Source: CAD feature listing. Evaluate the final solid. Frame: model axes, mm. Face numbers are marked on the shaded views. A direction names the side the tool comes from. Round coordinates to 2 decimals unless told otherwise and drop trailing zeros. Loops run counter-clockwise (first coordinate to the right, second up) from the corner with the lowest first, then second, coordinate; pieces in that order, holes last. Notation, with made-up numbers: (15, 49) -> (40, 49) arc R16 ccw to (40, 66) -> close; hole circle Ø3 at (-8, 50). An arc over 180 degrees is marked (long way). Return JSON: item names as keys, results as strings. Group by question number.
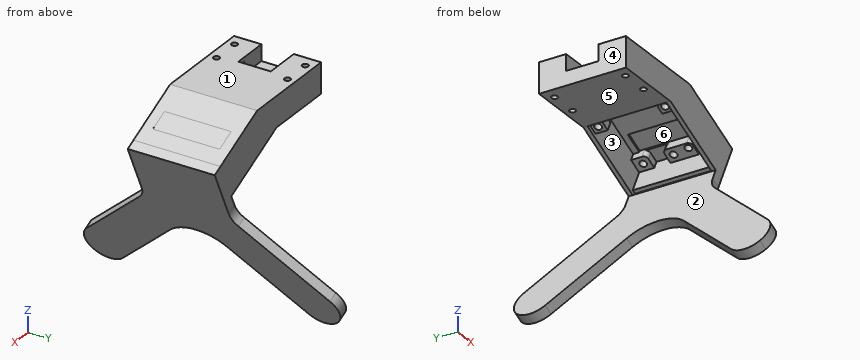
```python
from build123d import *

# Parameters (mm, degrees)
AUFSATZ_LINEAR_AUSTRAGEN1_DEPTH      = 43
AUFSATZ_LINEAR_AUSTRAGEN2_DEPTH      = 5
SCHNITT_LINEAR_AUSTRAGEN1_REACH      = 157.451
SKIZZE3_R                            = 1.5
SKIZZE4_W                            = 8
SKIZZE4_H                            = 16
SCHNITT_LINEAR_AUSTRAGEN2_DEPTH      = 18
SKIZZE5_W                            = 30
SKIZZE5_H                            = 39
SCHNITT_LINEAR_AUSTRAGEN3_DEPTH      = 18
SKIZZE6_W                            = 7
SKIZZE6_H                            = 7.5
SKIZZE6_H_2                          = 14
SKIZZE6_H_3                          = 5.5
AUFSATZ_LINEAR_AUSTRAGEN3_DEPTH      = 4
VERRUNDUNG1_R                        = 2
F_3_4_3_4_DURCHMESSER_BOHRUNG1_D     = 3.4
F_3_4_3_4_DURCHMESSER_BOHRUNG1_DEPTH = 4
SKIZZE10_W                           = 10
SKIZZE10_H                           = 33
SCHNITT_LINEAR_AUSTRAGEN4_DEPTH      = 1
SKIZZE11_W                           = 10
SKIZZE11_H                           = 33
SCHNITT_LINEAR_AUSTRAGEN5_DEPTH      = 0.001
SCHNITT_LINEAR_AUSTRAGEN7_DEPTH      = 39
SKIZZE15_W                           = 10.432594073
SKIZZE15_H                           = 24
SCHNITT_LINEAR_AUSTRAGEN10_DEPTH     = 16
SKIZZE16_W                           = 2.1
SKIZZE16_H                           = 39
SCHNITT_LINEAR_AUSTRAGEN11_DEPTH     = 2
VERRUNDUNG2_R                        = 20
VERRUNDUNG3_R                        = 10
SKIZZE17_W                           = 6
SKIZZE17_H                           = 6
AUFSATZ_LINEAR_AUSTRAGEN4_DEPTH      = 5
FASE1_SIZE                           = 6
F_3_4_3_4_DURCHMESSER_BOHRUNG2_D     = 3.4
F_3_4_3_4_DURCHMESSER_BOHRUNG2_DEPTH = 5
F_3_4_3_4_DURCHMESSER_BOHRUNG2_TIP   = 1.021463052


with BuildPart() as part:
    # Skizze1 → Aufsatz-Linear austragen1 (new body)
    with BuildSketch(Plane(origin=(0, 0, 0), x_dir=(1, 0, 0), z_dir=(0, 1, 0))):
        Polygon((0, 0), (50, 0), (78.641941074, 13.355956467), (70.189575839, 31.482112208), (34.843572145, 15), (0, 15), align=None)
    extrude(amount=AUFSATZ_LINEAR_AUSTRAGEN1_DEPTH)

    # Skizze2 → Aufsatz-Linear austragen2 (add)
    with BuildSketch(Plane(origin=(69.711631316, 0, -32.507067545), x_dir=(-0.4226182617407004, 0, -0.9063077870366495), z_dir=(0.9063077870366495, 0, -0.4226182617407004))):
        Polygon((-21.130913087, 43), (8.869086913, 43), (54.544231126, 88.675144213), (68.686366749, 74.533008589), (15.65335816, 21.5), (68.686366749, -31.533008589), (54.544231126, -45.675144213), (8.869086913, 0), (-21.130913087, 0), align=None)
    extrude(amount=AUFSATZ_LINEAR_AUSTRAGEN2_DEPTH)

    # Skizze3 → Schnitt-Linear austragen1 (cut, up to next)
    with BuildSketch(Plane.XY, mode=Mode.PRIVATE) as schnitt_linear_austragen1_sk1:
        with Locations((6, 39)):
            Circle(SKIZZE3_R)
    schnitt_linear_austragen1_tool1 = extrude(schnitt_linear_austragen1_sk1.sketch, amount=-SCHNITT_LINEAR_AUSTRAGEN1_REACH, mode=Mode.PRIVATE) & part.part
    # Skizze3 → Schnitt-Linear austragen1 (cut, up to next)
    with BuildSketch(Plane.XY, mode=Mode.PRIVATE) as schnitt_linear_austragen1_sk2:
        with Locations((20, 39)):
            Circle(SKIZZE3_R)
    schnitt_linear_austragen1_tool2 = extrude(schnitt_linear_austragen1_sk2.sketch, amount=-SCHNITT_LINEAR_AUSTRAGEN1_REACH, mode=Mode.PRIVATE) & part.part
    # Skizze3 → Schnitt-Linear austragen1 (cut, up to next)
    with BuildSketch(Plane.XY, mode=Mode.PRIVATE) as schnitt_linear_austragen1_sk3:
        with Locations((6, 4)):
            Circle(SKIZZE3_R)
    schnitt_linear_austragen1_tool3 = extrude(schnitt_linear_austragen1_sk3.sketch, amount=-SCHNITT_LINEAR_AUSTRAGEN1_REACH, mode=Mode.PRIVATE) & part.part
    # Skizze3 → Schnitt-Linear austragen1 (cut, up to next)
    with BuildSketch(Plane.XY, mode=Mode.PRIVATE) as schnitt_linear_austragen1_sk4:
        with Locations((20, 4)):
            Circle(SKIZZE3_R)
    schnitt_linear_austragen1_tool4 = extrude(schnitt_linear_austragen1_sk4.sketch, amount=-SCHNITT_LINEAR_AUSTRAGEN1_REACH, mode=Mode.PRIVATE) & part.part
    add(schnitt_linear_austragen1_tool1.solids().sort_by_distance((6, 39, 0))[0], mode=Mode.SUBTRACT)
    add(schnitt_linear_austragen1_tool2.solids().sort_by_distance((20, 39, 0))[0], mode=Mode.SUBTRACT)
    add(schnitt_linear_austragen1_tool3.solids().sort_by_distance((6, 4, 0))[0], mode=Mode.SUBTRACT)
    add(schnitt_linear_austragen1_tool4.solids().sort_by_distance((20, 4, 0))[0], mode=Mode.SUBTRACT)

    # Skizze4 → Schnitt-Linear austragen2 (cut)
    with BuildSketch(Plane.ZY):
        with Locations((-4, 21.5)):
            Rectangle(SKIZZE4_W, SKIZZE4_H)
    extrude(amount=-SCHNITT_LINEAR_AUSTRAGEN2_DEPTH, mode=Mode.SUBTRACT)

    # Skizze5 → Schnitt-Linear austragen3 (cut)
    with BuildSketch(Plane(origin=(0.477944523, 0, 1.024955337), x_dir=(-0.9063077870366492, 0, 0.4226182617407011), z_dir=(-0.4226182617407011, 0, -0.9063077870366492))):
        with Locations((-60.918274689, 21.5)):
            Rectangle(SKIZZE5_W, SKIZZE5_H)
    extrude(amount=-SCHNITT_LINEAR_AUSTRAGEN3_DEPTH, mode=Mode.SUBTRACT)

    # Skizze6 → Aufsatz-Linear austragen3 (add)
    with BuildSketch(Plane(origin=(8.085073234, 0, 17.338495504), x_dir=(-0.9063077870366492, 0, 0.42261826174070133), z_dir=(-0.42261826174070133, 0, -0.9063077870366492))):
        with Locations((-72.418274689, 37.25)):
            Rectangle(SKIZZE6_W, SKIZZE6_H)
        with Locations((-72.418274689, 18.5)):
            Rectangle(SKIZZE6_W, SKIZZE6_H_2)
        with Locations((-72.418274689, 4.75)):
            Rectangle(SKIZZE6_W, SKIZZE6_H_3)
    extrude(amount=AUFSATZ_LINEAR_AUSTRAGEN3_DEPTH)

    # Verrundung1
    verrundung1_edges = [part.edges().sort_by_distance(p)[0] for p in [
        (69.701005731, 33.5, -13.600241521),
        (69.701005731, 11.5, -13.600241521),
        (69.701005731, 25.5, -13.600241521),
        (69.701005731, 7.5, -13.600241521),
    ]]
    fillet(verrundung1_edges, radius=VERRUNDUNG1_R)

    # Ø3.4 (3.4) Durchmesser Bohrung1
    with Locations(Plane(origin=(6.394600187, 0, 13.713264356), x_dir=(-0.906307787036649, 0, 0.4226182617407016), z_dir=(-0.4226182617407016, 0, -0.906307787036649))):
        with Locations((-72.418274689, 37), (-72.418274689, 22), (-71.418274689, 14.1), (-71.418274689, 5)):
            Hole(F_3_4_3_4_DURCHMESSER_BOHRUNG1_D / 2, depth=F_3_4_3_4_DURCHMESSER_BOHRUNG1_DEPTH)

    # Skizze10 → Schnitt-Linear austragen4 (cut)
    with BuildSketch(Plane(origin=(8.085073234, 0, 17.338495504), x_dir=(-0.9063077870366492, 0, 0.42261826174070133), z_dir=(-0.42261826174070133, 0, -0.9063077870366492))):
        with Locations((-63.918274689, 21.5)):
            Rectangle(SKIZZE10_W, SKIZZE10_H)
    extrude(amount=-SCHNITT_LINEAR_AUSTRAGEN4_DEPTH, mode=Mode.SUBTRACT)

    # Skizze11 → Schnitt-Linear austragen5 (cut)
    with BuildSketch(Plane(origin=(8.930309758, 0, 19.151111078), x_dir=(0.9063077870366492, 0, -0.42261826174070133), z_dir=(0.42261826174070133, 0, 0.9063077870366492))):
        with Locations((63.918274689, 21.5)):
            Rectangle(SKIZZE11_W, SKIZZE11_H)
    extrude(amount=-SCHNITT_LINEAR_AUSTRAGEN5_DEPTH, mode=Mode.SUBTRACT)

    # Skizze12 → Schnitt-Linear austragen7 (cut)
    with BuildSketch(Plane(origin=(0, 2, 0), x_dir=(1, 0, 0), z_dir=(0, 1, 0))):
        Polygon((49.701163152, 2.067405927), (42.094034441, 18.380946094), (34.843572145, 15), (34.843572145, 12.5), (29.343572145, 12.5), (29.343572145, 2.067405927), align=None)
    extrude(amount=SCHNITT_LINEAR_AUSTRAGEN7_DEPTH, mode=Mode.SUBTRACT)

    # Skizze15 → Schnitt-Linear austragen10 (cut)
    with BuildSketch(Plane(origin=(29.343572145, 0, 0), x_dir=(0, 0, -1), z_dir=(1, 0, 0))):
        with Locations((7.283702963, 21.5)):
            Rectangle(SKIZZE15_W, SKIZZE15_H)
    extrude(amount=-SCHNITT_LINEAR_AUSTRAGEN10_DEPTH, mode=Mode.SUBTRACT)

    # Skizze16 → Schnitt-Linear austragen11 (cut)
    with BuildSketch(Plane(origin=(68.805323529, 0, -32.084449283), x_dir=(0.42261826174070133, 0, 0.9063077870366492), z_dir=(-0.9063077870366492, 0, 0.42261826174070133))):
        with Locations((2.180913087, 21.5)):
            Rectangle(SKIZZE16_W, SKIZZE16_H)
    extrude(amount=-SCHNITT_LINEAR_AUSTRAGEN11_DEPTH, mode=Mode.SUBTRACT)

    # Verrundung2
    verrundung2_edges = [part.edges().sort_by_distance(p)[0] for p in [
        (65.362005767, 21.5, -47.750373594),
    ]]
    fillet(verrundung2_edges, radius=VERRUNDUNG2_R)

    # Verrundung3
    verrundung3_edges = [part.edges().sort_by_distance(p)[0] for p in [
        (68.229162689, 43, -41.601735733),
        (68.229162689, 0, -41.601735733),
        (42.949287863, 74.533008589, -95.814602248),
        (48.926012637, 88.675144213, -82.997474607),
        (48.926012637, -45.675144213, -82.997474607),
        (42.949287863, -31.533008589, -95.814602248),
    ]]
    fillet(verrundung3_edges, radius=VERRUNDUNG3_R - 0.0001)  # a hair under: the kernel refuses the full size

    # Skizze17 → Aufsatz-Linear austragen4 (add)
    with BuildSketch(Plane(origin=(1.323181047, 0, 2.837570911), x_dir=(-0.9063077870366492, 0, 0.4226182617407011), z_dir=(-0.4226182617407011, 0, -0.9063077870366492))):
        with Locations((-40.918274689, 38)):
            Rectangle(SKIZZE17_W, SKIZZE17_H)
        with Locations((-40.918274689, 5)):
            Rectangle(SKIZZE17_W, SKIZZE17_H)
    extrude(amount=-AUFSATZ_LINEAR_AUSTRAGEN4_DEPTH)

    # Fase1
    fase1_edges = [part.edges().sort_by_distance(p)[0] for p in [
        (40.520823338, 2, -9.923700276),
        (40.520823338, 41, -9.923700276),
    ]]
    chamfer(fase1_edges, length=FASE1_SIZE - 0.0001)  # a hair under: the kernel refuses the full size

    # Ø3.4 (3.4) Durchmesser Bohrung2
    with Locations(Plane(origin=(1.323181047, 0, 2.837570911), x_dir=(-0.9063077870366492, 0, 0.4226182617407014), z_dir=(-0.42261826174070133, 0, -0.906307787036649))):
        with Locations((-40.918274689, 38), (-40.918274689, 5)):
            Hole(F_3_4_3_4_DURCHMESSER_BOHRUNG2_D / 2, depth=F_3_4_3_4_DURCHMESSER_BOHRUNG2_DEPTH)
            with Locations((0, 0, -(F_3_4_3_4_DURCHMESSER_BOHRUNG2_DEPTH + F_3_4_3_4_DURCHMESSER_BOHRUNG2_TIP / 2))):  # 118° drill point
                Cone(0, F_3_4_3_4_DURCHMESSER_BOHRUNG2_D / 2, F_3_4_3_4_DURCHMESSER_BOHRUNG2_TIP, mode=Mode.SUBTRACT)


solid = part.part
```
(1) Cut plane B-B (x = 9.5). Return loops of the section in (y, z).
(2) Ray query, line 1 (Y direction, x = 20, z = -11); line 2 (Y direction, x = 6, z = -5); line 3 (Y direction, x = 35, z = -6). Return the intervals inside material, ascending.
(3) Cut plane D-D (z = -49). Return loops of the section in (x, y), and give its area (3 significant figures).
(4) Cut plane A-A (x = 20). Return loops of the section in (y, z).
(5) Mould query, pull axis Z, two halves, no side actions, for the marked faces 4, 5 and 6. Classes: released by +Z, released by -Z, zero draft, split by the parting line, or undercut.
(6) Cut plane C-C (y = 50). Return loops of the section in (x, z).
(7) Set-up query: the marked faces 1, 2 and 3. Return all of +Z, -Z, +X, -X, +Y, -Y with unobstructed straight access to the full face (end or side cutting, diameter ignored); none if empty.
(8) Pin query (flat end, axial travel): pin 1 (1.7 mm diameter, centred on x = 72.5, z = -15, fed in from -Y); pin 2 (3.5 mm diameter, centred on x = 68, z = -8, fed in from +Y); pin 3 (2 mm diameter, centred on y = 5, z = -7.5, fed in from +X). Return the tip coordinate at first contact, or that it passes through.
Answers follow:
{
 "1": {"outline": "(0, -15) -> (43, -15) -> (43, 0) -> (29.5, 0) -> (29.5, -8) -> (13.5, -8) -> (13.5, 0) -> (0, 0) -> close"},
 "2": {"line 1": "0 to 2.5, 5.5 to 9.5, 33.5 to 37.5, 40.5 to 43", "line 2": "0 to 2.5, 5.5 to 13.5, 29.5 to 37.5, 40.5 to 43", "line 3": "0 to 2, 41 to 43"},
 "3": {"outline": "(62.02, -9.33) -> (67.54, -7) -> (67.54, 50) -> (62.02, 52.33) -> close", "area": "327 mm^2"},
 "4": {"outline": "(0, -15) -> (2.5, -15) -> (2.5, 0) -> (0, 0) -> close; (5.5, -15) -> (37.5, -15) -> (37.5, 0) -> (5.5, 0) -> close; (40.5, -15) -> (43, -15) -> (43, 0) -> (40.5, 0) -> close; hole (9.5, -12.5) -> (33.5, -12.5) -> (33.5, -2.07) -> (9.5, -2.07) -> close"},
 "5": {"face 4": "zero draft", "face 5": "released by -Z", "face 6": "undercut"},
 "6": {"outline": "(51.05, -72.52) -> (55.58, -74.64) -> (67.54, -49) -> (63.01, -46.89) -> close"},
 "7": {"face 1": "+Z, +X, -X, +Y, -Y", "face 2": "-X, +Y, -Y", "face 3": "none"},
 "8": {"pin 1": "y = 0", "pin 2": "y = 43", "pin 3": "x = 68.23"}
}
